```python
from build123d import *

# Parameters (mm, degrees)
SKETCH1_R               = 7.5565
BOSS_EXTRUDE1_DEPTH     = 8.89
SKETCH2_R               = 7.5565
SKETCH2_R_2             = 3.3
BOSS_EXTRUDE2_DEPTH     = 0.635
SKETCH3_W               = 1.979009817
SKETCH3_H               = 3.81
SKETCH3_W_2             = 2.256055482
CUT_EXTRUDE1_DEPTH      = 8.5565
CUT_EXTRUDE1_DEPTH_BACK = 8.5565


with BuildPart() as part:
    # Sketch1 → Boss-Extrude1 (new body)
    with BuildSketch(Plane(origin=(0, 0, 0), x_dir=(1, 0, 0), z_dir=(0, 1, 0))):
        Circle(SKETCH1_R)
        Polygon((-2.915618859, 5.05), (-5.831237719, 0), (-2.915618859, -5.05), (2.915618859, -5.05), (5.831237719, 0), (2.915618859, 5.05), align=None, mode=Mode.SUBTRACT)
    extrude(amount=BOSS_EXTRUDE1_DEPTH)

    # Sketch2 → Boss-Extrude2 (add)
    with BuildSketch(Plane.XZ):
        Circle(SKETCH2_R)
        Circle(SKETCH2_R_2, mode=Mode.SUBTRACT)
    extrude(amount=BOSS_EXTRUDE2_DEPTH)

    # Sketch3 → Cut-Extrude1 (cut, two sides)
    with BuildSketch(Plane(origin=(0, 0, 0), x_dir=(0, 0, -1), z_dir=(1, 0, 0))) as cut_extrude1_sk:
        with Locations((-7.212504909, 7.62)):
            Rectangle(SKETCH3_W, SKETCH3_H)
        with Locations((7.351027741, 7.62)):
            Rectangle(SKETCH3_W_2, SKETCH3_H)
    extrude(amount=CUT_EXTRUDE1_DEPTH, mode=Mode.SUBTRACT)
    extrude(cut_extrude1_sk.sketch, amount=-CUT_EXTRUDE1_DEPTH_BACK, mode=Mode.SUBTRACT)


solid = part.part
```
The model under review builds one solid part; all positions refer to its coordinate system, in mm. A direction names the side the tool comes from. Coordinates: 2 decimals unless noted, no trailing zeros. Order: outer loops, then holes, each group sorted by start corner. A loop starts at its lowest first (then second) coordinate and runs counter-clockwise, first axis right, second up. Notation, with made-up numbers: (83.25, 1) -> (96.25, 1) arc R25 cw to (96.25, 26) -> close; hole circle Ø6 at (41.25, 35). An arc over 180 degrees is marked (long way). Answer in a Markdown table with one row per item. Add a question column.
Item 1: To check wall thickness, follow probe 1 along Z at (x, y) = (0, -0.5); probe 2 along Z at (x, y) = (-2, 5.75); probe 3 along X at (y, z) = (4.75, 2.5). State the ranges of each line that lie inside material, in increasing order.
Item 2: We need section A-A on y = 0.5. Write out the cut boundary in (x, z), plus the area to 3 significant figures.
Item 3: Mouldability with a two-part tool opening along Z and no side actions: class faces 4 (the cylindrical face through (-7.55, 3.14, 0.33)), 5 (the flat face through (0, 4, 5.05)), 6 (the flat face through (0, 5.715, 7)) as +Z half, -Z half, draft (parallel to the pull), parting line (faces both ways), or undercut.
Item 4: We need section C-C on z = 3.75. Write out the cut boundary in (x, y) (3 decimals), plus the area to 3 significant figures.
Item 5: Machinability: for faces 1 (the flat face through (0, 4, -5.05)), 2 (the flat face through (0, 7, -6.223)), 3 (the flat face through (0, 7, 6.223)), which of the approach directions +Z, -Z, +X, -X, +Y, -Y give a long, thin tool a straight path to every point of the face, cutting with its end or side? Answer none if there is none.
Item 6: Clearance check with flat-ended pins moving along their axes: pin 1 (7.5 mm diameter, centred on x = 0, z = 0, fed in from -Y) (3 decimals); pin 2 (2.5 mm diameter, centred on x = -0.5, y = 7.5, fed in from -Z); pin 3 (1.5 mm diameter, centred on x = 1, y = 3.5, fed in from +Z); pin 4 (2 mm diameter, centred on x = 4.5, y = 6.5, fed in from -Z). State where each tip first meets the part, or that it passes through.
Item 7: We need section D-D on y = 7.5. Write out the cut boundary in (x, z).
Final values:
| question | item | result |
|---|---|---|
| 1 | probe 1 | z = -7.56 to -3.3, 3.3 to 7.56 |
| 1 | probe 2 | z = -6.22 to -5.05, 5.05 to 6.22 |
| 1 | probe 3 | x = -7.13 to -4.39, 4.39 to 7.13 |
| 2 | outline | circle Ø15.11 at (0, 0); hole (-5.83, 0) -> (-2.92, -5.05) -> (2.92, -5.05) -> (5.83, 0) -> (2.92, 5.05) -> (-2.92, 5.05) -> close |
| 2 | area | 91.0 mm2 |
| 3 | face 4 | parting line |
| 3 | face 5 | undercut |
| 3 | face 6 | draft |
| 4 | outline | (-6.56, -0.635) -> (6.56, -0.635) -> (6.56, 8.89) -> (3.666, 8.89) -> (3.666, 0) -> (-3.666, 0) -> (-3.666, 8.89) -> (-6.56, 8.89) -> close |
| 4 | area | 59.8 mm2 |
| 5 | face 1 | +Y |
| 5 | face 2 | -Z, +X, -X, +Y |
| 5 | face 3 | +Z, +X, -X, +Y |
| 6 | pin 1 | stops at y = -0.635 |
| 6 | pin 2 | stops at z = -6.22 |
| 6 | pin 3 | stops at z = 7.55 |
| 6 | pin 4 | stops at z = -6.48 |
| 7 | outline | (-4.29, -6.22) -> (4.29, -6.22) arc R7.56 ccw to (4.29, 6.22) -> (-4.29, 6.22) arc R7.56 ccw to start; hole (-5.83, 0) -> (-2.92, -5.05) -> (2.92, -5.05) -> (5.83, 0) -> (2.92, 5.05) -> (-2.92, 5.05) -> close |
